```python
from build123d import *

# Parameters (mm, degrees)
SKETCH1_W           = 60
SKETCH1_H           = 41
SKETCH1_R           = 5.25
SKETCH1_R_2         = 2
BOSS_EXTRUDE1_DEPTH = 20
SKETCH2_R           = 3
CUT_EXTRUDE1_DEPTH  = 55.598534779


with BuildPart() as part:
    # Sketch1 → Boss-Extrude1 (new body)
    with BuildSketch(Plane.XY):
        with Locations((0, -5.5)):
            Rectangle(SKETCH1_W, SKETCH1_H)
        Circle(SKETCH1_R, mode=Mode.SUBTRACT)
        with Locations((0, 8)):
            Circle(SKETCH1_R_2, mode=Mode.SUBTRACT)
        with Locations((8, 0)):
            Circle(SKETCH1_R_2, mode=Mode.SUBTRACT)
        with Locations((0, -8)):
            Circle(SKETCH1_R_2, mode=Mode.SUBTRACT)
        with Locations((-8, 0)):
            Circle(SKETCH1_R_2, mode=Mode.SUBTRACT)
    extrude(amount=BOSS_EXTRUDE1_DEPTH)

    # Sketch2 → Cut-Extrude1 (cut, through all)
    with BuildSketch(Plane(origin=(0, 15, 0), x_dir=(1, 0, 0), z_dir=(0, 1, 0))):
        with Locations(Location((-20, -10, 0), (0, 0, 270))):
            Circle(SKETCH2_R)
        with Locations(Location((20, -10, 0), (0, 0, 90))):
            Circle(SKETCH2_R)
    extrude(amount=-CUT_EXTRUDE1_DEPTH, mode=Mode.SUBTRACT)


solid = part.part
```
Verification items for the finished model (mm, model axes). Round coordinates to 2 decimals unless told otherwise and drop trailing zeros. Order: outer loops, then holes, each group sorted by start corner. A loop starts at its lowest first (then second) coordinate and runs counter-clockwise, first axis right, second up. Notation, with made-up numbers: (82, -12) -> (90, -12) arc R21 cw to (90, 17) -> close; hole circle Ø1 at (81, -21.5). An arc over 180 degrees is marked (long way). Put each result on its own line as item: value. Start each with the question number.
(1) Section check C-C (x = 20). Enter the section's corners in (y, z).
(2) Section check D-D (y = -8). Enter the section's corners in (x, z), then the cut area to 3 significant figures.
(3) Material ranges on line 1 along Y through (x, z) = (0, 12.5); line 2 along X through (y, z) = (-3.5, 10); line 3 along Y through (x, z) = (8, 14.5), recorded low to high.
(4) Section check A-A (y = 0). Enter the section's corners in (x, z).
(5) Draft check along X on faces 1 (the face through (0, 15, 10)), 2 (the face through (-30, -6, 10)), 3 (the face through (0, -6, 10)). Enter one of: +X half, -X half, draft (parallel to the pull), parting line (faces both ways), or undercut.
(6) Section check B-B (z = 10). Enter the section's corners in (x, y).
Completed:
1. outline: (-26, 0) -> (15, 0) -> (15, 7) -> (-26, 7) -> close; (-26, 13) -> (15, 13) -> (15, 20) -> (-26, 20) -> close
2. outline: (-30, 0) -> (-2, 0) -> (-2, 20) -> (-30, 20) -> close; (2, 0) -> (30, 0) -> (30, 20) -> (2, 20) -> close; hole circle Ø6 at (-20, 10); hole circle Ø6 at (20, 10)
2. area: 1,060 mm2
3. line 1: y = -26 to -10, -6 to -5.25, 5.25 to 6, 10 to 15
3. line 2: x = -30 to -23, -17 to -3.91, 3.91 to 17, 23 to 30
3. line 3: y = -26 to -2, 2 to 15
4. outline: (-30, 0) -> (-10, 0) -> (-10, 20) -> (-30, 20) -> close; (-6, 0) -> (-5.25, 0) -> (-5.25, 20) -> (-6, 20) -> close; (5.25, 0) -> (6, 0) -> (6, 20) -> (5.25, 20) -> close; (10, 0) -> (30, 0) -> (30, 20) -> (10, 20) -> close; hole circle Ø6 at (-20, 10); hole circle Ø6 at (20, 10)
5. face 1: draft
5. face 2: -X half
5. face 3: undercut
6. outline: (-30, -26) -> (-23, -26) -> (-23, 15) -> (-30, 15) -> close; (-17, -26) -> (17, -26) -> (17, 15) -> (-17, 15) -> close; (23, -26) -> (30, -26) -> (30, 15) -> (23, 15) -> close; hole circle Ø4 at (-8, 0); hole circle Ø10.5 at (0, 0); hole circle Ø4 at (0, -8); hole circle Ø4 at (0, 8); hole circle Ø4 at (8, 0)
